from build123d import *

# Parameters (mm, degrees)
SKETCH_1_R      = 1.5
SKETCH_1_W      = 18.5
SKETCH_1_H      = 18.5
SKETCH_1_W_2    = 19
SKETCH_1_H_2    = 17
SKETCH_1_H_3    = 19
EXTRUDE_1_DEPTH = 2


with BuildPart() as part:
    # 草图1 → 凸台-拉伸1 (new body)
    with BuildSketch(Plane(origin=(0, 0, 0), x_dir=(1, 0, 0), z_dir=(0, 1, 0))):
        with BuildLine():
            Line((10, 0), (136.884360712, 0))
            ThreePointArc((136.884360712, 0), (137.900113715, -0.277140216), (138.634360712, -1.031754163))
            Line((138.634360712, -1.031754163), (139.429147615, -2.468245837))
            ThreePointArc((139.429147615, -2.468245837), (140.163394612, -3.222859784), (141.179147615, -3.5))
            Line((141.179147615, -3.5), (143.5, -3.5))
            Line((143.5, -3.5), (166.5, -3.5))
            Line((166.5, -3.5), (168.820852385, -3.5))
            ThreePointArc((168.820852385, -3.5), (169.836605388, -3.222859784), (170.570852385, -2.468245837))
            Line((170.570852385, -2.468245837), (171.365639288, -1.031754163))
            ThreePointArc((171.365639288, -1.031754163), (172.099886285, -0.277140216), (173.115639288, 0))
            Line((173.115639288, 0), (300, 0))
            ThreePointArc((300, 0), (307.071067812, -2.928932188), (310, -10))
            Line((310, -10), (310, -210))
            ThreePointArc((310, -210), (307.071067812, -217.071067812), (300, -220))
            Line((300, -220), (10, -220))
            ThreePointArc((10, -220), (2.928932188, -217.071067812), (0, -210))
            Line((0, -210), (0, -10))
            ThreePointArc((0, -10), (2.928932188, -2.928932188), (10, 0))
        make_face()
        with Locations(Location((14, -14, 0), (0, 0, 270))):
            Circle(SKETCH_1_R, mode=Mode.SUBTRACT)
        with Locations(Location((14, -206, 0), (0, 0, 270))):
            Circle(SKETCH_1_R, mode=Mode.SUBTRACT)
        with Locations(Location((296, -206, 0), (0, 0, 270))):
            Circle(SKETCH_1_R, mode=Mode.SUBTRACT)
        with Locations(Location((296, -12.28568254, 0), (0, 0, 270))):
            Circle(SKETCH_1_R, mode=Mode.SUBTRACT)
        with Locations(Location((155, -206, 0), (0, 0, 270))):
            Circle(SKETCH_1_R, mode=Mode.SUBTRACT)
        with Locations(Location((175, -14, 0), (0, 0, 270))):
            Circle(SKETCH_1_R, mode=Mode.SUBTRACT)
        with Locations(Location((135, -14, 0), (0, 0, 270))):
            Circle(SKETCH_1_R, mode=Mode.SUBTRACT)
        with Locations(Location((296, -110, 0), (0, 0, 270))):
            Circle(SKETCH_1_R, mode=Mode.SUBTRACT)
        with Locations(Location((14, -110, 0), (0, 0, 270))):
            Circle(SKETCH_1_R, mode=Mode.SUBTRACT)
        with Locations(Location((155, -110, 0), (0, 0, 270))):
            Circle(SKETCH_1_R, mode=Mode.SUBTRACT)
        with Locations(Location((72, -110, 0), (0, 0, 270))):
            Circle(SKETCH_1_R, mode=Mode.SUBTRACT)
        with Locations(Location((72, -168.903225806, 0), (0, 0, 270))):
            Circle(SKETCH_1_R, mode=Mode.SUBTRACT)
        with Locations(Location((72, -51.096774194, 0), (0, 0, 270))):
            Circle(SKETCH_1_R, mode=Mode.SUBTRACT)
        with Locations(Location((42, -168.903225806, 0), (0, 0, 270))):
            Circle(SKETCH_1_R, mode=Mode.SUBTRACT)
        with Locations(Location((102, -168.903225806, 0), (0, 0, 270))):
            Circle(SKETCH_1_R, mode=Mode.SUBTRACT)
        with Locations(Location((238, -110, 0), (0, 0, 270))):
            Circle(SKETCH_1_R, mode=Mode.SUBTRACT)
        with Locations(Location((238, -168.903225806, 0), (0, 0, 270))):
            Circle(SKETCH_1_R, mode=Mode.SUBTRACT)
        with Locations(Location((268, -168.903225806, 0), (0, 0, 270))):
            Circle(SKETCH_1_R, mode=Mode.SUBTRACT)
        with Locations(Location((208, -168.903225806, 0), (0, 0, 270))):
            Circle(SKETCH_1_R, mode=Mode.SUBTRACT)
        with Locations(Location((246, -39, 0), (0, 0, 270))):
            Circle(SKETCH_1_R, mode=Mode.SUBTRACT)
        with Locations(Location((198, -39, 0), (0, 0, 270))):
            Circle(SKETCH_1_R, mode=Mode.SUBTRACT)
        with Locations(Location((110, -70, 0), (0, 0, 270))):
            Circle(SKETCH_1_R, mode=Mode.SUBTRACT)
        with Locations(Location((38, -51.096774194, 0), (0, 0, 270))):
            Circle(SKETCH_1_R, mode=Mode.SUBTRACT)
        with Locations(Location((198, -110, 0), (0, 0, 270))):
            Circle(SKETCH_1_R, mode=Mode.SUBTRACT)
        with Locations(Location((143.5, -90, 0), (0, 0, 270))):
            Circle(SKETCH_1_R, mode=Mode.SUBTRACT)
        with Locations((38, -24)):
            Rectangle(SKETCH_1_W, SKETCH_1_H, mode=Mode.SUBTRACT)
        with Locations((62, -24)):
            Rectangle(SKETCH_1_W, SKETCH_1_H, mode=Mode.SUBTRACT)
        with Locations((86, -24)):
            Rectangle(SKETCH_1_W, SKETCH_1_H, mode=Mode.SUBTRACT)
        with Locations((110, -24)):
            Rectangle(SKETCH_1_W, SKETCH_1_H, mode=Mode.SUBTRACT)
        with Locations((198, -24)):
            Rectangle(SKETCH_1_W, SKETCH_1_H, mode=Mode.SUBTRACT)
        with Locations((222, -24)):
            Rectangle(SKETCH_1_W, SKETCH_1_H, mode=Mode.SUBTRACT)
        with Locations((246, -24)):
            Rectangle(SKETCH_1_W, SKETCH_1_H, mode=Mode.SUBTRACT)
        with Locations((270, -24)):
            Rectangle(SKETCH_1_W, SKETCH_1_H, mode=Mode.SUBTRACT)
        with Locations((89, -53)):
            Rectangle(SKETCH_1_W_2, SKETCH_1_H_2, mode=Mode.SUBTRACT)
        with Locations((84, -77)):
            Rectangle(SKETCH_1_W_2, SKETCH_1_H_2, mode=Mode.SUBTRACT)
        with Locations((106, -90)):
            Rectangle(SKETCH_1_W_2, SKETCH_1_H_2, mode=Mode.SUBTRACT)
        with Locations((58, -80)):
            Rectangle(SKETCH_1_W_2, SKETCH_1_H_2, mode=Mode.SUBTRACT)
        with Locations((36, -97)):
            Rectangle(SKETCH_1_W_2, SKETCH_1_H_2, mode=Mode.SUBTRACT)
        with Locations((114, -130)):
            Rectangle(SKETCH_1_W_2, SKETCH_1_H_3, mode=Mode.SUBTRACT)
        with Locations((145, -138)):
            Rectangle(SKETCH_1_W_2, SKETCH_1_H_3, mode=Mode.SUBTRACT)
        with Locations((190, -130)):
            Rectangle(SKETCH_1_W_2, SKETCH_1_H_3, mode=Mode.SUBTRACT)
        with Locations((173, -85)):
            Rectangle(SKETCH_1_W_2, SKETCH_1_H_2, mode=Mode.SUBTRACT)
        with Locations((190, -66)):
            Rectangle(SKETCH_1_W_2, SKETCH_1_H_2, mode=Mode.SUBTRACT)
        with Locations((198, -90)):
            Rectangle(SKETCH_1_W_2, SKETCH_1_H_2, mode=Mode.SUBTRACT)
        with Locations((215, -58)):
            Rectangle(SKETCH_1_W_2, SKETCH_1_H_2, mode=Mode.SUBTRACT)
        with Locations((222, -84)):
            Rectangle(SKETCH_1_W_2, SKETCH_1_H_2, mode=Mode.SUBTRACT)
        with Locations((241, -58)):
            Rectangle(SKETCH_1_W_2, SKETCH_1_H_2, mode=Mode.SUBTRACT)
        with Locations((247, -84)):
            Rectangle(SKETCH_1_W_2, SKETCH_1_H_2, mode=Mode.SUBTRACT)
        with Locations((266, -66)):
            Rectangle(SKETCH_1_W_2, SKETCH_1_H_2, mode=Mode.SUBTRACT)
    extrude(amount=EXTRUDE_1_DEPTH)


solid = part.part
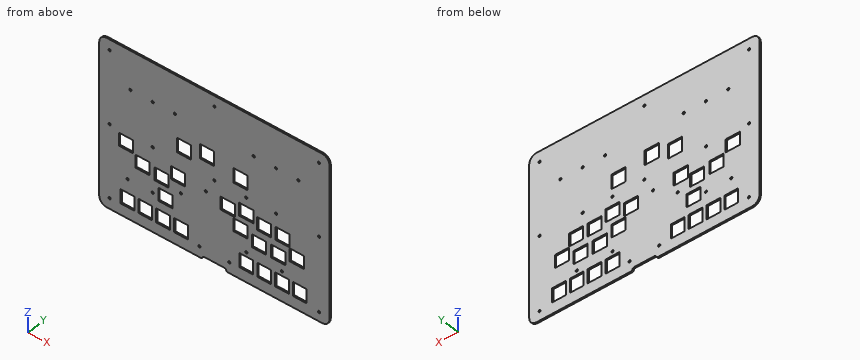
Could you check a few things on this model? Use its own coordinates, in mm. Give positions to 0.01 mm unless a question says otherwise; leave off trailing zeros.
Item 1: I'm going to push a flat-ended pin straight in: pin 1 (5 mm diameter, centred on x = 238, z = 110, fed in from +Y). Where does the tip first touch, or does it pass through?
Item 2: I need wall thicknesses on line 1 (Z direction, x = 97.5, y = 0.9); line 2 (Z direction, x = 143.5, y = 0.95); line 3 (X direction, y = 1.9, z = 96.5). Which ranges of each line are inside material? Lowest first, please.
Item 3: If we section it at A-A, the plane y = 0.7: Count the separate pieces of the cut face and the enclosed holes in it, plus the area to 3 significant figures.
Values:
1. pin 1: stops at y = 2
2. line 1: z = 0 to 44.5, 61.5 to 81.5, 98.5 to 220
2. line 2: z = 3.5 to 88.5, 91.5 to 128.5, 147.5 to 220
2. line 3: x = 0 to 26.5, 45.5 to 96.5, 115.5 to 188.5, 207.5 to 310
3. separate pieces: 1
3. enclosed holes: 49
3. area: 59,800 mm2
